Geometry check sheet. Reference: the model listing, model coordinates, mm. Give positions to 0.01 mm unless a question says otherwise; leave off trailing zeros. Loops run counter-clockwise (first coordinate to the right, second up) from the corner with the lowest first, then second, coordinate; pieces in that order, holes last.
```python
from build123d import *

# Parameters (mm, degrees)
F1_DEPTH = 1.08
F3_D     = 13.5


with BuildPart() as f1:
    # F0 (on Front) → F1 (new body)
    with BuildSketch(Plane.XZ):
        with BuildLine():
            Line((-45, 0), (-1, 0))
            ThreePointArc((-1, 0), (-0.292893, 0.292893), (0, 1))
            Line((0, 1), (0, 56))
            ThreePointArc((0, 56), (-0.292893, 56.707107), (-1, 57))
            Line((-1, 57), (-45, 57))
            ThreePointArc((-45, 57), (-48.535534, 55.535534), (-50, 52))
            Line((-50, 52), (-50, 5))
            ThreePointArc((-50, 5), (-48.535534, 1.464466), (-45, 0))
        make_face()
    extrude(amount=F1_DEPTH)

    # F3 (through all)
    with Locations(Plane.XZ.offset(1.08)):
        with Locations((-22, 44.5), (-22.069119, 12.5)):
            Hole(F3_D / 2)


solid = f1.part
```
1) Sectioned sample at C-C on x = -22. Enter the section's corners in (y, z).
2) Sectioned sample at B-B on z = 12.5. Enter the section's corners in (x, y).
3) Mould release check, pull along X, two halves, no side actions. Record for faces 1 (the cylindrical face through (-48.5, -0.53, 55.57)), 2 (the flat face through (-25, -1.08, 29)), 3 (the cylindrical face through (-20.61, -0.53, 5.91)): +X half, -X half, draft (parallel to the pull), parting line (faces both ways), or undercut.
4) Sectioned sample at D-D on z = 39.5. Enter the section's corners in (x, y), plus the area to 3 significant figures.
5) Sectioned sample at A-A on y = -0.3. Enter the section's corners in (x, z).
6) Scan lines: line 1 along Z through (x, y) = (-22, -0.6); line 2 along Z through (x, y) = (-24, -0.7); line 3 along X through (y, z) = (-0.5, 50). Record each from-to range of solid material in increasing order.
Determined:
1. outline: (-1.08, 0) - (0, 0) - (0, 5.75) - (-1.08, 5.75) - close; (-1.08, 19.25) - (0, 19.25) - (0, 37.75) - (-1.08, 37.75) - close; (-1.08, 51.25) - (0, 51.25) - (0, 57) - (-1.08, 57) - close
2. outline: (-50, -1.08) - (-28.82, -1.08) - (-28.82, 0) - (-50, 0) - close; (-15.32, -1.08) - (0, -1.08) - (0, 0) - (-15.32, 0) - close
3. face 1: -X half
3. face 2: draft
3. face 3: undercut
4. outline: (-50, -1.08) - (-26.53, -1.08) - (-26.53, 0) - (-50, 0) - close; (-17.47, -1.08) - (0, -1.08) - (0, 0) - (-17.47, 0) - close
4. area: 44.2 mm2
5. outline: (-50, 5) arc R5 ccw to (-45, 0) - (-1, 0) arc R1 ccw to (0, 1) - (0, 56) arc R1 ccw to (-1, 57) - (-45, 57) arc R5 ccw to (-50, 52) - close; hole circle Ø13.5 at (-22.07, 12.5); hole circle Ø13.5 at (-22, 44.5)
6. line 1: z = 0 to 5.75, 19.25 to 37.75, 51.25 to 57
6. line 2: z = 0 to 6.03, 18.97 to 38.05, 50.95 to 57
6. line 3: x = -50 to -25.91, -18.09 to 0
